Read the model definition and answer for the solid it produces. Units are mm, in the model's axes. Face numbers are marked on the shaded views. A direction names the side the tool comes from. Coordinates: 2 decimals unless noted, no trailing zeros. Write each loop counter-clockwise with the first axis right and the second up, starting at its lowest first coordinate (ties: lowest second). Pieces come first, ordered by that corner, then holes. Notation, with made-up numbers: (65.5, -39.5) -> (110.5, -39.5) arc R22 cw to (110.5, -14.5) -> close; hole circle Ø2 at (63.5, -37.75). An arc over 180 degrees is marked (long way). Write item = value, one per line. Start each with the question number.
1) A tool of negligible diameter and unlimited length cuts with its end or side. For the marked faces 1 and 2, from which of +Z, -Z, +X, -X, +Y, -Y can it reach the whole face along a straight path? Write none if from no direction.
2) Section A-A (x = 0) is taken. Determine the outline of the cut face in (y, z).
3) For a pull along Z with two mould halves and no side action, classify the marked faces 3, 4 and 5 as released by +Z, released by -Z, zero draft, split by the parting line, or undercut.
4) Flat-ended cylindrical pins translate along their axes: pin 1 Ø8 at (x, z) = (0, 0) entering from -Y; pin 2 Ø1.5 at (x, z) = (0, 5.5) entering from +Y; pin 3 Ø3 at (x, z) = (0, 0) entering from +Y; pin 4 Ø2 at (x, y) = (-2, 1.5) entering from +Z. Find the tip coordinate at first contact, or state that the pin passes through.
5) Section B-B (z = 0) is taken. Determine the outline of the cut face in (x, y), plus the area to 3 significant figures.
6) Section D-D (z = -3) is taken. Determine the outline of the cut face in (x, y), plus the area to 3 significant figures.
7) Section C-C (x = -3) is taken. Determine the outline of the cut face in (y, z).
8) Find the intervals of material crossed by line 1 along X through (y, z) = (0.3, 3); line 2 along Y through (x, z) = (-5, 6.75), in increasing order. Write a range as from..to.
from build123d import *

# Parameters (mm, degrees)
SKETCH1_R           = 9.8
BOSS_EXTRUDE1_DEPTH = 1.1
SKETCH2_R           = 3.35
BOSS_EXTRUDE2_DEPTH = 3.1
SKETCH3_R           = 2.5
CUT_EXTRUDE1_DEPTH  = 2.5
CUT_EXTRUDE2_REACH  = 3.7
SKETCH4_R           = 1
SKETCH5_R           = 2
CUT_EXTRUDE3_DEPTH  = 0.5
SKETCH6_R           = 0.5
CUT_EXTRUDE4_DEPTH  = 5.2
CIRPATTERN1_COUNT   = 4


with BuildPart() as part:
    # Sketch1 → Boss-Extrude1 (new body)
    with BuildSketch(Plane(origin=(0, 0, 0), x_dir=(1, 0, 0), z_dir=(0, 1, 0))):
        Circle(SKETCH1_R)
    extrude(amount=BOSS_EXTRUDE1_DEPTH)

    # Sketch2 → Boss-Extrude2 (add)
    with BuildSketch(Plane(origin=(0, 1.1, 0), x_dir=(1, 0, 0), z_dir=(0, 1, 0))):
        Circle(SKETCH2_R)
    extrude(amount=BOSS_EXTRUDE2_DEPTH)

    # Sketch3 → Cut-Extrude1 (cut)
    with BuildSketch(Plane(origin=(0, 4.2, 0), x_dir=(1, 0, 0), z_dir=(0, 1, 0))):
        Circle(SKETCH3_R)
    extrude(amount=-CUT_EXTRUDE1_DEPTH, mode=Mode.SUBTRACT)

    # Sketch4 → Cut-Extrude2 (cut, up to next)
    with BuildSketch(Plane(origin=(0, 1.7, 0), x_dir=(1, 0, 0), z_dir=(0, 1, 0)), mode=Mode.PRIVATE) as cut_extrude2_sk1:
        Circle(SKETCH4_R)
    cut_extrude2_tool1 = extrude(cut_extrude2_sk1.sketch, amount=-CUT_EXTRUDE2_REACH, mode=Mode.PRIVATE) & part.part
    add(cut_extrude2_tool1.solids().sort_by_distance((0, 1.7, 0))[0], mode=Mode.SUBTRACT)

    # Sketch5 → Cut-Extrude3 (cut)
    with BuildSketch(Plane.XZ):
        Circle(SKETCH5_R)
    extrude(amount=-CUT_EXTRUDE3_DEPTH, mode=Mode.SUBTRACT)

    # Sketch6 → Cut-Extrude4 (cut, through all)
    with BuildSketch(Plane.XZ):
        with Locations((-3, 7.5)):
            Circle(SKETCH6_R)
        with Locations((0, 7.5)):
            Circle(SKETCH6_R)
        with Locations((3, 7.5)):
            Circle(SKETCH6_R)
    cut_extrude4 = extrude(amount=-CUT_EXTRUDE4_DEPTH, mode=Mode.SUBTRACT)

    # CirPattern1: Cut-Extrude4 ×4 about axis
    cirpattern1_axis = Axis((0, 0, 0), (0, 1, 0))
    for i in range(1, CIRPATTERN1_COUNT):
        add(cut_extrude4.rotate(cirpattern1_axis, i * 360 / CIRPATTERN1_COUNT), mode=Mode.SUBTRACT)


solid = part.part
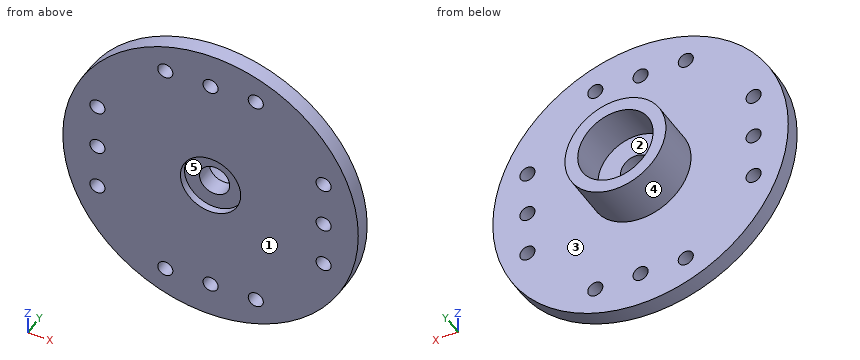
Answer key:
q1.face_1 = +Z, -Z, +X, -X, -Y
q1.face_2 = +Y
q2.outline = (0, -9.8) -> (1.1, -9.8) -> (1.1, -8) -> (0, -8) -> close; (0, -7) -> (1.1, -7) -> (1.1, -3.35) -> (4.2, -3.35) -> (4.2, -2.5) -> (1.7, -2.5) -> (1.7, -1) -> (0.5, -1) -> (0.5, -2) -> (0, -2) -> close; (0, 2) -> (0.5, 2) -> (0.5, 1) -> (1.7, 1) -> (1.7, 2.5) -> (4.2, 2.5) -> (4.2, 3.35) -> (1.1, 3.35) -> (1.1, 7) -> (0, 7) -> close; (0, 8) -> (1.1, 8) -> (1.1, 9.8) -> (0, 9.8) -> close
q3.face_3 = zero draft
q3.face_4 = split by the parting line
q3.face_5 = undercut
q4.pin_1 = 0
q4.pin_2 = 1.1
q4.pin_3 = 1.7
q4.pin_4 = 9.74
q5.outline = (-9.8, 0) -> (-8, 0) -> (-8, 1.1) -> (-9.8, 1.1) -> close; (-7, 0) -> (-2, 0) -> (-2, 0.5) -> (-1, 0.5) -> (-1, 1.7) -> (-2.5, 1.7) -> (-2.5, 4.2) -> (-3.35, 4.2) -> (-3.35, 1.1) -> (-7, 1.1) -> close; (1, 0.5) -> (2, 0.5) -> (2, 0) -> (7, 0) -> (7, 1.1) -> (3.35, 1.1) -> (3.35, 4.2) -> (2.5, 4.2) -> (2.5, 1.7) -> (1, 1.7) -> close; (8, 0) -> (9.8, 0) -> (9.8, 1.1) -> (8, 1.1) -> close
q5.area = 23.2 mm^2
q6.outline = (-9.33, 0) -> (-8, 0) -> (-8, 1.1) -> (-9.33, 1.1) -> close; (-7, 0) -> (7, 0) -> (7, 1.1) -> (1.49, 1.1) -> (1.49, 4.2) -> (-1.49, 4.2) -> (-1.49, 1.1) -> (-7, 1.1) -> close; (8, 0) -> (9.33, 0) -> (9.33, 1.1) -> (8, 1.1) -> close
q6.area = 27.6 mm^2
q7.outline = (0, -9.33) -> (1.1, -9.33) -> (1.1, -8) -> (0, -8) -> close; (0, -7) -> (1.1, -7) -> (1.1, -1.49) -> (4.2, -1.49) -> (4.2, 1.49) -> (1.1, 1.49) -> (1.1, 7) -> (0, 7) -> close; (0, 8) -> (1.1, 8) -> (1.1, 9.33) -> (0, 9.33) -> close
q8.line_1 = -9.33..-8, -7..7, 8..9.33
q8.line_2 = 0..1.1
